The listing builds one solid part. Answer for the finished solid, in the listing's coordinates (mm). A direction names the side the tool comes from. Coordinates: 2 decimals unless noted, no trailing zeros. Order: outer loops, then holes, each group sorted by start corner. A loop starts at its lowest first (then second) coordinate and runs counter-clockwise, first axis right, second up.
from build123d import *

# Parameters (mm, degrees)
BOSS_EXTRUDE1_DEPTH     = 9.525
SKETCH2_W               = 17.78
SKETCH2_H               = 177.8
BOSS_EXTRUDE2_DEPTH     = 2.794
F_1_4_CLEARANCE_HOLE1_D = 6.7564
F_1_4_CLEARANCE_HOLE2_D = 6.7564


with BuildPart() as part:
    # Sketch1 → Boss-Extrude1 (new, symmetric)
    with BuildSketch(Plane(origin=(0, 0, 0), x_dir=(1, 0, 0), z_dir=(0, 1, 0))):
        with BuildLine():
            Line((-76.2, 88.9), (-152.4, 88.9))
            Line((-152.4, 88.9), (-152.4, -88.9))
            Line((-152.4, -88.9), (152.4, -88.9))
            Line((152.4, -88.9), (152.4, 88.9))
            Line((152.4, 88.9), (76.2, 88.9))
            ThreePointArc((76.2, 88.9), (0, 28.883239197), (-76.2, 88.9))
        make_face()
    extrude(amount=BOSS_EXTRUDE1_DEPTH, both=True)

    # Sketch2 → Boss-Extrude2 (add, symmetric)
    with BuildSketch(Plane(origin=(0, 0, 0), x_dir=(1, 0, 0), z_dir=(0, 1, 0))):
        with Locations((-161.29, 0)):
            Rectangle(SKETCH2_W, SKETCH2_H)
        with Locations((161.29, 0)):
            Rectangle(SKETCH2_W, SKETCH2_H)
    extrude(amount=BOSS_EXTRUDE2_DEPTH, both=True)

    # 1/4 Clearance Hole1 (through all)
    with Locations(Plane(origin=(0, 2.794, 0), x_dir=(1, 0, 0), z_dir=(0, 1, 0))):
        with Locations((158.75, 63.5), (158.75, 25.4), (158.75, -25.4)):
            f_1_4_clearance_hole1 = Hole(F_1_4_CLEARANCE_HOLE1_D / 2)

    # Mirror1: 1/4 Clearance Hole1 across plane
    add(f_1_4_clearance_hole1.mirror(Plane(origin=(0, 0, 0), x_dir=(0, 0, 1), z_dir=(1, 0, 0))), mode=Mode.SUBTRACT)

    # 1/4 Clearance Hole2 (through all)
    with Locations(Plane(origin=(0, 9.525, 0), x_dir=(1, 0, 0), z_dir=(0, 1, 0))):
        with Locations((-127, -79.375), (-50.8, -79.375)):
            f_1_4_clearance_hole2 = Hole(F_1_4_CLEARANCE_HOLE2_D / 2)

    # Mirror2: 1/4 Clearance Hole2 across plane
    add(f_1_4_clearance_hole2.mirror(Plane(origin=(0, 0, 0), x_dir=(0, 0, 1), z_dir=(1, 0, 0))), mode=Mode.SUBTRACT)


solid = part.part
(1) Find section C-C on z = 57. Determine the outline of the cut face in (x, y) (3 decimals).
(2) Find section B-B on x = 127. Determine the outline of the cut face in (y, z) (3 decimals).
(3) Find the intervals of material crossed by probe 1 along Z at (x, y) = (-158.75, -1.1); probe 2 along Z at (x, y) = (-127, -2.75); probe 3 along Y at (x, z) = (-153, -5.5), in increasing order.
(4) Given pin 1 Ø1 at (x, y) = (-45.5, 6.5) entering from -Z; pin 2 Ø8 at (x, z) = (-158.75, 25.4) entering from -Y; pin 3 Ø5.5 at (y, z) = (-6.5, -33.5) entering from -X, each flat-ended and moving along its own axis, determine where each tip first touches the part or whether it passes through.
(5) Find section A-A on z = 25.4. Determine the outline of the cut face in (x, y) (3 decimals).
(6) A tool of negligible diameter and unlimited length cuts with its end or side. For faces 4 (the flat face through (152.4, -6, 1)), 5 (the flat face through (-161, -2.794, -1)), 6 (the flat face through (152.4, 6, 1)), 7 (the cylindrical face through (-157.2, 0, -60.5)), from which of +Z, -Z, +X, -X, +Y, -Y can it reach the whole face along a straight path? Write none if from no direction.
(7) The mould has two halves that part along X. Classify faces 1 (the flat face through (-2, 9.525, 19)), 2 (the cylindrical face through (-155.528, -0.039, 24.385)), 3 (the flat face through (-152.4, -6, -1)): pulls with the +X half, pulls with the -X half, needs draft (parallel to the pull), parting line crosses it, or undercut.
(8) Find section D-D on z = -63.5. Determine the outline of the cut face in (x, y) (3 decimals), then the cut area to 3 significant figures.
Resolved:
1. outline: (-170.18, -2.794) - (-152.4, -2.794) - (-152.4, -9.525) - (152.4, -9.525) - (152.4, -2.794) - (170.18, -2.794) - (170.18, 2.794) - (152.4, 2.794) - (152.4, 9.525) - (-152.4, 9.525) - (-152.4, 2.794) - (-170.18, 2.794) - close
2. outline: (-9.525, -88.9) - (9.525, -88.9) - (9.525, 75.997) - (-9.525, 75.997) - close; (-9.525, 82.753) - (9.525, 82.753) - (9.525, 88.9) - (-9.525, 88.9) - close
3. probe 1: z = -88.9 to -66.88, -60.12 to -28.78, -22.02 to 22.02, 28.78 to 88.9
3. probe 2: z = -88.9 to 76, 82.75 to 88.9
3. probe 3: y = -2.79 to 2.79
4. pin 1: stops at z = -43.8
4. pin 2: stops at y = -2.79
4. pin 3: stops at x = -152.4
5. outline: (-170.18, -2.794) - (-162.128, -2.794) - (-162.128, 2.794) - (-170.18, 2.794) - close; (-155.372, -2.794) - (-152.4, -2.794) - (-152.4, -9.525) - (152.4, -9.525) - (152.4, -2.794) - (155.372, -2.794) - (155.372, 2.794) - (152.4, 2.794) - (152.4, 9.525) - (-152.4, 9.525) - (-152.4, 2.794) - (-155.372, 2.794) - close; (162.128, -2.794) - (170.18, -2.794) - (170.18, 2.794) - (162.128, 2.794) - close
6. face 4: +Z, -Z, +X, -Y
6. face 5: +Z, -Z, -X, -Y
6. face 6: +Z, -Z, +X, +Y
6. face 7: +Y, -Y
7. face 1: needs draft
7. face 2: undercut
7. face 3: pulls with the -X half
8. outline: (-170.18, -2.794) - (-162.128, -2.794) - (-162.128, 2.794) - (-170.18, 2.794) - close; (-155.372, -2.794) - (-152.4, -2.794) - (-152.4, -9.525) - (-65.026, -9.525) - (-65.026, 9.525) - (-152.4, 9.525) - (-152.4, 2.794) - (-155.372, 2.794) - close; (65.026, -9.525) - (152.4, -9.525) - (152.4, -2.794) - (155.372, -2.794) - (155.372, 2.794) - (152.4, 2.794) - (152.4, 9.525) - (65.026, 9.525) - close; (162.128, -2.794) - (170.18, -2.794) - (170.18, 2.794) - (162.128, 2.794) - close
8. area: 3,450 mm2
